The listing builds one solid part. Answer for the finished solid, in the listing's coordinates (mm). Give positions to 0.01 mm unless a question says otherwise; leave off trailing zeros. Loops run counter-clockwise (first coordinate to the right, second up) from the corner with the lowest first, then second, coordinate; pieces in that order, holes last.
Item 1: Consider line 1 along X through (y, z) = (-9, 1.25). Determine where the line is inside the solid, lowest interval first.
Item 2: Each of these flat-tipped pins is pushed along its axis until it touches: pin 1 Ø2 at (y, z) = (18, 4.5) entering from +X; pin 2 Ø2.5 at (y, z) = (-7, 2) entering from -X. Where does it stop, or does it pass through?
Item 3: Section B-B, the plane y = -6 is taken. Give the vertices of the cut face in (x, z), and give its area (3 significant figures).
Item 4: Section A-A, the plane z = 2.8 is taken. Give the vertices of the cut face in (x, y), and give its area (3 significant figures).
from build123d import *

# Parameters (mm, degrees)
F0_W     = 5.116921
F0_H     = 5.349506
F0_W_2   = 5.349502
F1_DEPTH = 4.826


with BuildPart() as f1:
    # F0 (on Top) → F1 (new body)
    with BuildSketch(Plane.XY):
        Polygon((62.56596, 39.772414), (-38.842063, 39.772414), (-38.842063, 34.422908), (-38.842063, -39.539825), (62.56596, -39.539825), (62.56596, 34.422908), align=None)
        with Locations((-41.400523, 37.097661)):
            Rectangle(F0_W, F0_H)
        with Locations((65.240711, 37.097661)):
            Rectangle(F0_W_2, F0_H)
    extrude(amount=F1_DEPTH)


solid = f1.part
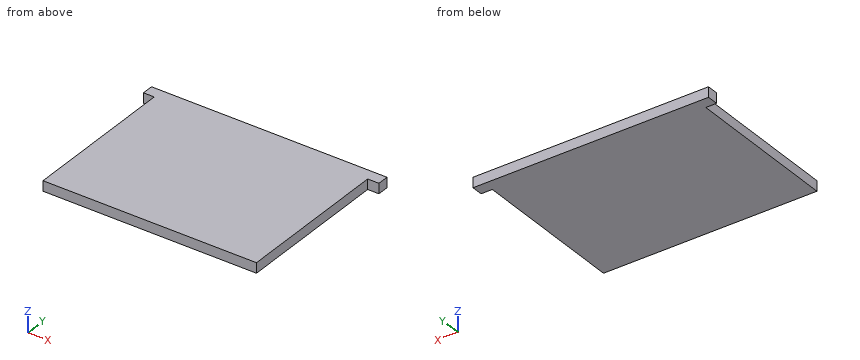
Worked answers:
1. line 1: x = -38.84 to 62.57
2. pin 1: stops at x = 62.57
2. pin 2: stops at x = -38.84
3. outline: (-38.84, 0) - (62.57, 0) - (62.57, 4.83) - (-38.84, 4.83) - close
3. area: 489 mm2
4. outline: (-43.96, 34.42) - (-38.84, 34.42) - (-38.84, -39.54) - (62.57, -39.54) - (62.57, 34.42) - (67.92, 34.42) - (67.92, 39.77) - (-43.96, 39.77) - close
4. area: 8,100 mm2
